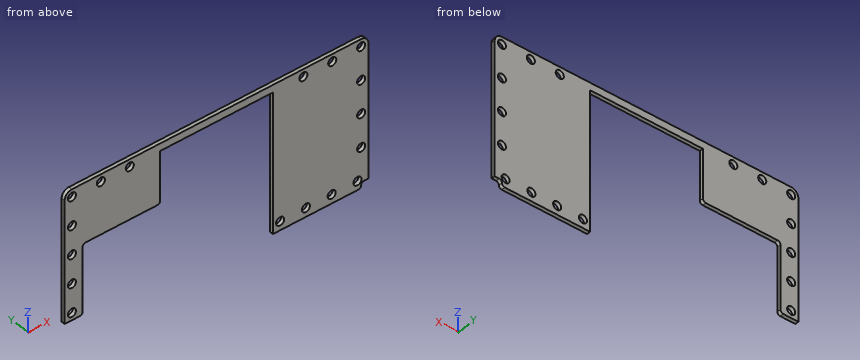
from build123d import *

# Parameters (mm, degrees)
BOSS_EXTRUDE1_DEPTH     = 1.5875
SKETCH2_R               = 1.778
CUT_EXTRUDE1_DEPTH      = 1
CUT_EXTRUDE1_DEPTH_BACK = 2.5875
FILLET1_R               = 1.27
SKETCH3_W               = 34.036
SKETCH3_H               = 12.7
CUT_EXTRUDE2_DEPTH      = 1
CUT_EXTRUDE2_DEPTH_BACK = 2.5875
FILLET2_R               = 1.27


with BuildPart() as part:
    # Sketch1 → Boss-Extrude1 (new body)
    with BuildSketch(Plane(origin=(0, 0, 0), x_dir=(1, 0, 0), z_dir=(0, 1, 0))):
        with BuildLine():
            Line((-66.675, 3.175), (-66.675, 55.209357386))
            Line((-66.675, 55.209357386), (-58.801, 55.209357386))
            Line((-58.801, 55.209357386), (-58.801, 36.83))
            Line((-58.801, 36.83), (-24.765, 36.83))
            Line((-24.765, 36.83), (-24.765, 3.175))
            Line((-24.765, 3.175), (24.765, 3.175))
            Line((24.765, 3.175), (24.765, 62.865))
            Line((24.765, 62.865), (62.23, 62.865))
            ThreePointArc((62.23, 62.865), (63.128025612, 62.493025612), (63.5, 61.595))
            ThreePointArc((63.5, 61.595), (63.871974388, 60.696974388), (64.77, 60.325))
            Line((64.77, 60.325), (66.675, 60.325))
            Line((66.675, 60.325), (66.675, 3.175))
            ThreePointArc((66.675, 3.175), (65.74506403, 0.92993597), (63.5, 0))
            Line((63.5, 0), (-63.5, 0))
            ThreePointArc((-63.5, 0), (-65.74506403, 0.92993597), (-66.675, 3.175))
        make_face()
    extrude(amount=BOSS_EXTRUDE1_DEPTH)

    # Sketch2 → Cut-Extrude1 (cut, two sides)
    with BuildSketch(Plane(origin=(0, 1.5875, 0), x_dir=(-1, 0, 0), z_dir=(0, 1, 0))) as cut_extrude1_sk:
        with Locations((63.5, -3.175)):
            Circle(SKETCH2_R)
        with Locations((50.8, -3.175)):
            Circle(SKETCH2_R)
        with Locations((38.1, -3.175)):
            Circle(SKETCH2_R)
        with Locations((-38.1, -3.175)):
            Circle(SKETCH2_R)
        with Locations((-50.8, -3.175)):
            Circle(SKETCH2_R)
        with Locations((-63.5, -3.175)):
            Circle(SKETCH2_R)
        with Locations((63.5, -15.389839347)):
            Circle(SKETCH2_R)
        with Locations((63.5, -27.604678693)):
            Circle(SKETCH2_R)
        with Locations((63.5, -39.81951804)):
            Circle(SKETCH2_R)
        with Locations((63.5, -52.034357386)):
            Circle(SKETCH2_R)
        with Locations((-63.5, -17.337603912)):
            Circle(SKETCH2_R)
        with Locations((-63.5, -31.500207823)):
            Circle(SKETCH2_R)
        with Locations((-63.5, -45.662811735)):
            Circle(SKETCH2_R)
        with Locations((-61.869746345, -59.055)):
            Circle(SKETCH2_R)
        with Locations((-50.559830897, -59.055)):
            Circle(SKETCH2_R)
        with Locations((-39.249915448, -59.055)):
            Circle(SKETCH2_R)
        with Locations((-27.94, -59.055)):
            Circle(SKETCH2_R)
    extrude(amount=CUT_EXTRUDE1_DEPTH, mode=Mode.SUBTRACT)
    extrude(cut_extrude1_sk.sketch, amount=-CUT_EXTRUDE1_DEPTH_BACK, mode=Mode.SUBTRACT)

    # Fillet1
    fillet1_edges = [part.edges().sort_by_distance(p)[0] for p in [
        (-58.801, 0.79375, -55.209357386),
        (-58.801, 0.79375, -36.83),
        (-24.765, 0.79375, -36.83),
    ]]
    fillet(fillet1_edges, radius=FILLET1_R)

    # Sketch3 → Cut-Extrude2 (cut, two sides)
    with BuildSketch(Plane(origin=(0, 1.5875, 0), x_dir=(1, 0, 0), z_dir=(0, 1, 0))) as cut_extrude2_sk:
        with Locations((-41.783, 31.75)):
            Rectangle(SKETCH3_W, SKETCH3_H)
    extrude(amount=CUT_EXTRUDE2_DEPTH, mode=Mode.SUBTRACT)
    extrude(cut_extrude2_sk.sketch, amount=-CUT_EXTRUDE2_DEPTH_BACK, mode=Mode.SUBTRACT)

    # Fillet2
    fillet2_edges = [part.edges().sort_by_distance(p)[0] for p in [
        (-24.765, 0.79375, -25.4),
        (-58.801, 0.79375, -25.4),
    ]]
    fillet(fillet2_edges, radius=FILLET2_R)


solid = part.part
Geometry check sheet. Reference: the model listing, model coordinates, mm. Round coordinates to 2 decimals unless told otherwise and drop trailing zeros. Order: outer loops, then holes, each group sorted by start corner. A loop starts at its lowest first (then second) coordinate and runs counter-clockwise, first axis right, second up. Notation, with made-up numbers: M 75.5,-33 L 114.5,-33 A36 ccw 114.5,1 Z; hole C -4,-37.75 d10. An arc over 180 degrees is marked long. Answer in a Markdown table with one row per item. Add a question column.
Item 1: Sectioned sample at C-C, the plane y = 0.3. State how many separate pieces and enclosed holes the cut face has, plus the area to 3 significant figures.
Item 2: Sectioned sample at D-D, the plane x = -15. Enter the section's corners in (y, z) (1 decimal), plus the area to 3 significant figures.
Item 3: Depth check by flat-ended pin: pin 1 Ø0.8 at (x, y) = (-39.5, 1) entering from -Z. Enter the tip coordinate at first touch or a pass-through.
Item 4: Sectioned sample at B-B, the plane x = 50.8. Enter the section's corners in (y, z) (1 decimal).
Item 5: Material ranges on L1, parallel to X at y = 1.55, z = -27.5 (3 decimals); L2, parallel to Z at x = -63.5, y = 1.1; L3, parallel to X at y = 0.85, z = -45.5 (3 decimals), recorded low to high. Write a range as [from, to].
Item 6: Sectioned sample at A-A, the plane x = -50.8. Enter the section's corners in (y, z).
Filled in:
| question | item | result |
|---|---|---|
| 1 | separate pieces | 1 |
| 1 | enclosed holes | 17 |
| 1 | area | 3,910 mm² |
| 2 | outline | M 0,-3.2 L 1.6,-3.2 L 1.6,0 L 0,0 Z |
| 2 | area | 5.04 mm² |
| 3 | pin 1 | stops at z = -25.4 |
| 4 | outline | M 0,-62.9 L 1.6,-62.9 L 1.6,-60.8 L 0,-60.8 Z; M 0,-57.3 L 1.6,-57.3 L 1.6,-5 L 0,-5 Z; M 0,-1.4 L 1.6,-1.4 L 1.6,0 L 0,0 Z |
| 5 | L1 | x = [-66.675, -65.275], [-61.725, -58.801], [24.765, 66.675] |
| 5 | L2 | z = [-55.21, -53.81], [-50.26, -41.6], [-38.04, -29.38], [-25.83, -17.17], [-13.61, -4.95], [-1.4, 0] |
| 5 | L3 | x = [-66.675, -58.801], [24.765, 61.729], [65.271, 66.675] |
| 6 | outline | M 0,-25.4 L 1.59,-25.4 L 1.59,-4.95 L 0,-4.95 Z; M 0,-1.4 L 1.59,-1.4 L 1.59,0 L 0,0 Z |
